Can you work these out from the model? Positions are in its coordinate system, mm. Coordinates: 2 decimals unless noted, no trailing zeros. Write each loop counter-clockwise with the first axis right and the second up, starting at its lowest first coordinate (ties: lowest second). Pieces come first, ordered by that corner, then holes. Notation, with made-up numbers: (-28, -14) -> (9, -14) arc R26 ccw to (9, 1) -> close; hole circle Ø11 at (23.25, 70.25). An arc over 180 degrees is marked (long way). Answer as CSV lines item,"result". Start each with the question number.
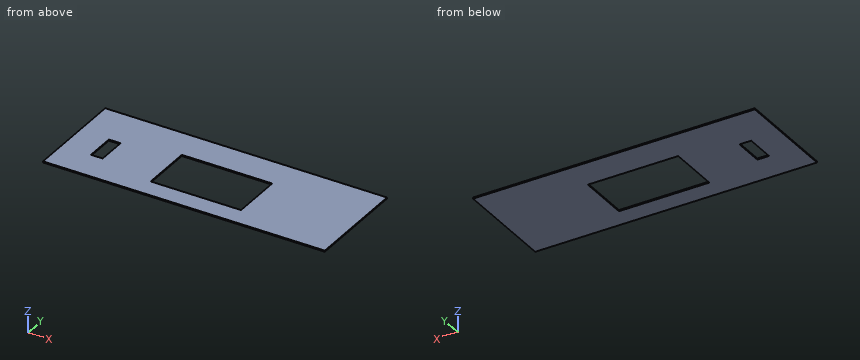
```python
from build123d import *

# Parameters (mm, degrees)
SKETCH1_W           = 480
SKETCH1_H           = 174
SKETCH1_W_2         = 154
SKETCH1_H_2         = 87
SKETCH1_W_3         = 20
SKETCH1_H_3         = 50
BOSS_EXTRUDE1_DEPTH = 2


with BuildPart() as part:
    # Sketch1 → Boss-Extrude1 (new body)
    with BuildSketch(Plane.XY):
        Rectangle(SKETCH1_W, SKETCH1_H)
        with Locations((0, -10)):
            Rectangle(SKETCH1_W_2, SKETCH1_H_2, mode=Mode.SUBTRACT)
        with Locations((-180, -10)):
            Rectangle(SKETCH1_W_3, SKETCH1_H_3, mode=Mode.SUBTRACT)
    extrude(amount=-BOSS_EXTRUDE1_DEPTH)


solid = part.part
```
Q1. I need wall thicknesses on L1, parallel to X at y = 12, z = -0.7; L2, parallel to Y at x = -55, z = -1.65; L3, parallel to X at y = -49, z = -0.85. Which ranges of each line are inside material? Lowest first, please.
Q2. Imagine slicing it at A-A (y = 23.5). Write out the boundary of the cut face in (x, z).
Q3. Imagine slicing it at B-B (x = -185.5). Write out the boundary of the cut face in (y, z), then the cut area to 3 significant figures.
Q4. Imagine slicing it at C-C (y = -26). Write out the boundary of the cut face in (x, z).
Q5. Imagine slicing it at D-D (z = -0.4). Write out the boundary of the cut face in (x, y), then the cut area to 3 significant figures.
Entries:
1,L1,"-240 to -190, -170 to -77, 77 to 240"
1,L2,"-87 to -53.5, 33.5 to 87"
1,L3,"-240 to -77, 77 to 240"
2,outline,"(-240, -2) -> (-77, -2) -> (-77, 0) -> (-240, 0) -> close; (77, -2) -> (240, -2) -> (240, 0) -> (77, 0) -> close"
3,outline,"(-87, -2) -> (-35, -2) -> (-35, 0) -> (-87, 0) -> close; (15, -2) -> (87, -2) -> (87, 0) -> (15, 0) -> close"
3,area,"248 mm2"
4,outline,"(-240, -2) -> (-190, -2) -> (-190, 0) -> (-240, 0) -> close; (-170, -2) -> (-77, -2) -> (-77, 0) -> (-170, 0) -> close; (77, -2) -> (240, -2) -> (240, 0) -> (77, 0) -> close"
5,outline,"(-240, -87) -> (240, -87) -> (240, 87) -> (-240, 87) -> close; hole (-190, -35) -> (-170, -35) -> (-170, 15) -> (-190, 15) -> close; hole (-77, -53.5) -> (77, -53.5) -> (77, 33.5) -> (-77, 33.5) -> close"
5,area,"69,100 mm2"
